Autodesk Inventor part; units mm, degrees
ref_plane "YZ Plane" through (0, 0, 0) normal (1, 0, 0) x (0, 1, 0)
ref_plane "XZ Plane" through (0, 0, 0) normal (0, 1, 0) x (-1, 0, 0)
ref_plane "XY Plane" through (0, 0, 0) normal (0, 0, 1) x (1, 0, 0)
sketch "Esquisse1" plane through (0, 0, 0) normal (0, 0, 1) x (1, 0, 0)
  line L0 (0, 0) -> (-71.5, 0)
  line L1 (-71.5, 0) -> (-71.5, 39)
  line L2 (-71.5, 39) -> (0, 39)
  line L3 (0, 39) -> (0, 0)
  dimension "d0" = 71.5
  dimension "d1" = 39
extrude "Extrusion1" add sketch "Esquisse1" along normal blind 5
sketch "Esquisse2" plane through (0, 0, 5) normal (0, 0, 1) x (1, 0, 0)
  line L0 (0, 39) -> (-71.5, 39)
  line L1 (-71.5, 39) -> (0, 0)
  line L2 (0, 0) -> (0, 39)
  line L3 (-71.5, 0) -> (0, 39)
  circle A0 centre (-35.75, 19.5) radius 5
  dimension "d4" = 10
extrude "Extrusion2" cut sketch "Esquisse2" against normal blind 5 contours A0 L1 L3 | L3 L1 A0 | L1 L3 A0 | A0 L3 L1
sketch "Esquisse3" plane through (-71.5, 0, 0) normal (-1, 0, 0) x (0, 0, 1)
  line L0 (0, 39) -> (5, 39)
  line L1 (5, 39) -> (54.4, 39)
  line L2 (54.4, 39) -> (54.4, 0)
  line L3 (54.4, 0) -> (5, 0)
  line L4 (5, 0) -> (5, 39)
  point P0 (0, 0)
  dimension "d7" = 49.4
extrude "Extrusion3" add sketch "Esquisse3" against normal blind 5
fillet "Congé1" radius 18 1 edges at (-69, 0, 54.4)
fillet "Congé2" radius 18 1 edges at (-69, 39, 54.4)
sketch "Esquisse4" plane through (-71.5, 0, 0) normal (-1, 0, 0) x (0, 0, 1)
  line L0 (36.4, 0) -> (5, 0)
  line L1 (5, 0) -> (54.4, 39)
  line L2 (5, 39) -> (5, 0)
  line L3 (5, 39) -> (54.4, 0)
  circle A0 centre (29.7, 19.5) radius 5
  point P0 (0, 0)
  dimension "d12" = 10
extrude "Extrusion4" add sketch "Esquisse4" along normal blind 10 contours A0 L3 L1 | L1 L3 A0 | L3 A0 L1 | L1 A0 L3
sketch "Esquisse5" plane through (0, 0, 0) normal (1, 0, 0) x (0, 0, -1)
  line L0 (-5, 0) -> (-81.9, 0)
  line L1 (-81.9, 0) -> (-81.9, 39)
  line L2 (-81.9, 39) -> (-5, 39)
  line L3 (-5, 39) -> (-5, 0)
  point P0 (0, 0)
  point P1 (-36.4, 39)
  dimension "d15" = 76.9
  dimension "d16" = 39
extrude "Extrusion5" add sketch "Esquisse5" against normal blind 5
fillet "Congé3" radius 10 1 edges at (-2.5, 39, 81.9)
fillet "Congé4" radius 10 1 edges at (-2.5, 0, 81.9)
sketch "Esquisse6" plane through (0, 0, 0) normal (1, 0, 0) x (0, 0, -1)
  line L0 (-60.501, 9.5) -> (-19.501, 9.5)
  line L1 (-19.501, 29.5) -> (-60.501, 29.5)
  circle A0 centre (-15.111, 14.5) radius 2.5
  circle A1 centre (-15.111, 24.5) radius 2.5
  circle A2 centre (-64.891, 14.5) radius 2.5
  circle A3 centre (-64.891, 24.5) radius 2.5
  line L2 (-19.501, 18.5) -> (-12.001, 18.5)
  line L3 (-12.001, 18.5) -> (-12.001, 20.5)
  line L4 (-12.001, 20.5) -> (-19.501, 20.5)
  line L5 (-60.501, 18.5) -> (-68.001, 18.5)
  line L6 (-68.001, 18.5) -> (-68.001, 20.5)
  line L7 (-68.001, 20.5) -> (-60.501, 20.5)
  line L8 (-19.501, 9.5) -> (-19.501, 18.5)
  line L9 (-19.501, 20.5) -> (-19.501, 29.5)
  line L10 (-60.501, 9.5) -> (-60.501, 18.5)
  line L11 (-60.501, 20.5) -> (-60.501, 29.5)
  line L12 (0, 0) -> (-71.9, 0)
  line L13 (0, 39) -> (-71.9, 39)
  line L14 (0, 39) -> (0, 0)
  point P0 (-29.706, 19.5075)
  dimension "d21" = 41
  dimension "d22" = 20
  dimension "d23" = 5
  dimension "d24" = 5
  dimension "d25" = 5
  dimension "d26" = 5
  dimension "d27" = 10
  dimension "d29" = 5
  dimension "d30" = 10
  dimension "d31" = 5
  dimension "d33" = 9
  dimension "d34" = 9
  dimension "d35" = 9
  dimension "d36" = 9
  dimension "d37" = 7.5
  dimension "d38" = 7.5
  dimension "d40" = 9.5
  dimension "d41" = 9.5
  dimension "d42" = 4.39
  dimension "d43" = 4.39
  dimension "d44" = 10.205
  dimension "d49" = 29.706
  dimension "d50" = 41
  dimension "d51" = 4.39
  dimension "d52" = 4.39
extrude "Extrusion6" cut sketch "Esquisse6" against normal blind 5
fillet "Congé5" radius 2 1 edges at (-66.5, 19.5, 5)
fillet "Congé6" radius 2 1 edges at (-5, 19.5, 5)
properties part number "ShoulderPart1" material "Plastique ABS"
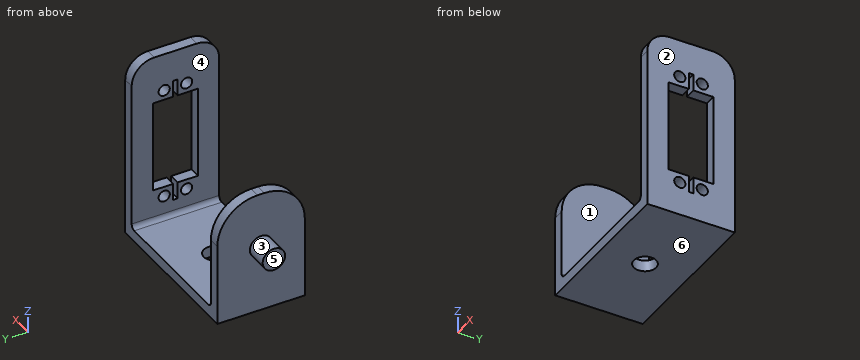
Geometry check sheet. Reference: the model listing, model coordinates, mm. Face numbers are marked on the shaded views. A direction names the side the tool comes from. Coordinates: 2 decimals unless noted, no trailing zeros. Order: outer loops, then holes, each group sorted by start corner. A loop starts at its lowest first (then second) coordinate and runs counter-clockwise, first axis right, second up. Notation, with made-up numbers: (67.25, -23) -> (116.25, -23) arc R24 cw to (116.25, 8) -> close; hole circle Ø11 at (54, -5.5). An arc over 180 degrees is marked (long way). Use a Markdown table: item, result. Add a question column.
1. Mould release check, pull along X, two halves, no side actions. Record for the marked faces 4, 5 and 6: pulls with the +X half, pulls with the -X half, needs draft (parallel to the pull), parting line crosses it, or undercut.
2. Cross-section at B-B (x = -35.75). Enter the section's corners in (y, z).
3. Cross-section at C-C (z = 29.7). Enter the section's corners in (x, y), and give its area (3 significant figures).
4. Set-up check for the marked faces 1, 2 and 3: record each of +Z, -Z, +X, -X, +Y, -Y from which the full face is reachable in a straight line by a thin tool's end or side.
5. Cross-section at A-A (y = 19.5). Enter the section's corners in (x, z).
6. Go/stop test with flat-tipped pins: pin 1 Ø3 at (x, y) = (-29.5, 34) entering from +Z; pin 2 Ø6 at (y, z) = (4.5, 57.5) entering from -X; pin 3 Ø0.9 at (x, y) = (-70, 20) entering from +Z. Record where each tip stops, or that it passes through.
7. Material ranges on L1, parallel to X at y = 12, z = 18; L2, parallel to X at y = 24, z = 30.5; L3, parallel to Z at x = -22.5, y = 27.5, recorded low to high.
8. Cross-section at D-D (y = 26). Enter the section's corners in (x, z), and give its area (3 significant figures).
Filled sheet:
| question | item | result |
|---|---|---|
| 1 | face 4 | undercut |
| 1 | face 5 | pulls with the -X half |
| 1 | face 6 | needs draft |
| 2 | outline | (0, 0) -> (14.5, 0) -> (14.5, 5) -> (0, 5) -> close; (24.5, 0) -> (39, 0) -> (39, 5) -> (24.5, 5) -> close |
| 3 | outline | (-81.5, 14.5) -> (-71.5, 14.5) -> (-71.5, 0) -> (-66.5, 0) -> (-66.5, 39) -> (-71.5, 39) -> (-71.5, 24.5) -> (-81.5, 24.5) -> close; (-5, 0) -> (0, 0) -> (0, 9.5) -> (-5, 9.5) -> close; (-5, 29.5) -> (0, 29.5) -> (0, 39) -> (-5, 39) -> close |
| 3 | area | 390 mm2 |
| 4 | face 1 | +Z, +Y, -Y |
| 4 | face 2 | +Z, -Z, +X, +Y, -Y |
| 4 | face 3 | -X |
| 5 | outline | (-81.5, 24.7) -> (-71.5, 24.7) -> (-71.5, 0) -> (-40.75, 0) -> (-40.75, 5) -> (-64.5, 5) arc R2 cw to (-66.5, 7) -> (-66.5, 54.4) -> (-71.5, 54.4) -> (-71.5, 34.7) -> (-81.5, 34.7) -> close; (-30.75, 0) -> (0, 0) -> (0, 12) -> (-5, 12) -> (-5, 7) arc R2 cw to (-7, 5) -> (-30.75, 5) -> close; (-5, 68) -> (0, 68) -> (0, 81.9) -> (-5, 81.9) -> close |
| 6 | pin 1 | z = 5 |
| 6 | pin 2 | x = -5 |
| 6 | pin 3 | z = 54.4 |
| 7 | L1 | -71.5 to -66.5, -5 to 0 |
| 7 | L2 | -81.5 to -66.5 |
| 7 | L3 | 0 to 5 |
| 8 | outline | (-71.5, 0) -> (0, 0) -> (0, 13.11) -> (-5, 13.11) -> (-5, 7) arc R2 cw to (-7, 5) -> (-64.5, 5) arc R2 cw to (-66.5, 7) -> (-66.5, 53.69) -> (-71.5, 53.69) -> close; (-5, 17.11) -> (0, 17.11) -> (0, 19.5) -> (-5, 19.5) -> close; (-5, 60.5) -> (0, 60.5) -> (0, 62.89) -> (-5, 62.89) -> close; (-5, 66.89) -> (0, 66.89) -> (0, 81.9) -> (-5, 81.9) -> close |
| 8 | area | 742 mm2 |
